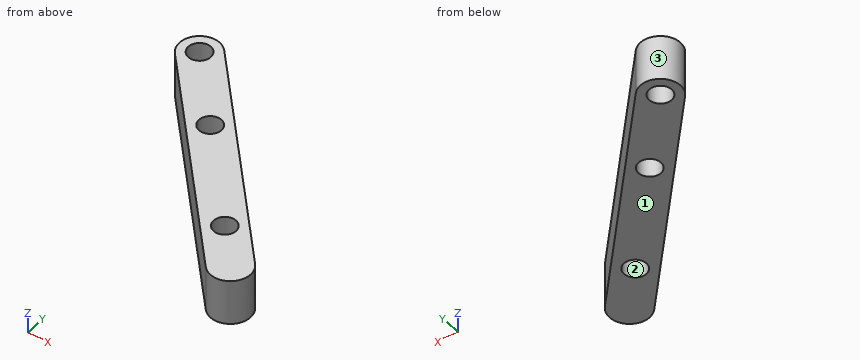
Autodesk Inventor part; units mm, degrees
ref_plane "YZ Plane" through (0, 0, 0) normal (1, 0, 0) x (0, 1, 0)
ref_plane "XZ Plane" through (0, 0, 0) normal (0, 1, 0) x (-1, 0, 0)
ref_plane "XY Plane" through (0, 0, 0) normal (0, 0, 1) x (1, 0, 0)
sketch "Sketch1" plane through (0, 0, 0) normal (0, 0, 1) x (1, 0, 0)
  circle A0 centre (20.6614, -0.7818) radius 2.25
  circle A1 centre (3.6717, 18.234) radius 2.25
  circle A2 centre (-8.6609, 32.0238) radius 2.25
  arc A3 (24.8863, -10.4155) -> (29.7342, -6.0856) centre (27.3102, -8.2505) ccw
  line L0 (27.3102, -8.2505) -> (-8.6609, 32.0238) construction
  line L1 (30.2936, -5.586) -> (-5.6776, 34.6883)
  line L2 (-11.6442, 29.3592) -> (24.3269, -10.9151)
  arc A4 (24.3269, -10.9151) -> (30.2936, -5.586) centre (27.3102, -8.2505) ccw
  arc A5 (-5.6776, 34.6883) -> (-11.6442, 29.3592) centre (-8.6609, 32.0238) ccw
  point P0 (0, 0)
  point P1 (9.3247, 11.8866)
  dimension "d0" = 8
extrude "Extrusion1" add sketch "Sketch1" along normal blind 9
scale "Scale1" factors (0.5, 0.5, 0.5) then translate (3.1707, 4.611, 2.25) bodies 1
properties part number "MassiveBone3"
The model under review builds one solid part; all positions refer to its coordinate system, in mm. Face numbers are marked on the shaded views. Coordinates: 2 decimals unless noted, no trailing zeros. Write each loop counter-clockwise with the first axis right and the second up, starting at its lowest first coordinate (ties: lowest second). Pieces come first, ordered by that corner, then holes. Notation, with made-up numbers: (28, -10.75) -> (58, -10.75) arc R18 ccw to (58, 9.25) -> close; hole circle Ø1 at (64, 31.25). An arc over 180 degrees is marked (long way). One line per item, written item: value. Start each with the question number.
Q1. The part is to be moulded in two halves that separate along Y. For the marked faces 1, 2 and 3, say which applies: +Y half, -Y half, draft (parallel to the pull), parting line (faces both ways), or undercut.
Q2. To check wall thickness, follow probe 1 along X at (y, z) = (20.5, 4.3); probe 2 along Y at (x, z) = (14.5, 4.95); probe 3 along Y at (x, z) = (13, 4.25). State the ranges of each line that lie inside material, in increasing order.
Q3. Add section A-A, the plane x = 4.25. Give the boundary of the cut face in (y, z), then the cut area to 3 significant figures.
Q4. Add section C-C, the plane y = 5. Give the boundary of the cut face in (x, z), then the cut area to 3 significant figures.
Q5. Add section D-D, the plane y = 0.5. Give the boundary of the cut face in (x, z), then the cut area to 3 significant figures.
Q6. Add section B-B, the plane z = 2.8. Count the separate pieces of the cut face and the enclosed holes in it, then the cut area to 3 significant figures.
Response:
1. face 1: draft
1. face 2: undercut
1. face 3: parting line
2. probe 1: -3.16 to -2.28, -0.04 to 1.63
2. probe 2: 0.09 to 3.7, 4.74 to 6.09
2. probe 3: 1.77 to 3.21, 5.23 to 7.77
3. outline: (11.56, 2.25) -> (12.9, 2.25) -> (12.9, 6.75) -> (11.56, 6.75) -> close; (14.56, 2.25) -> (17.57, 2.25) -> (17.57, 6.75) -> (14.56, 6.75) -> close
3. area: 19.5 mm²
4. outline: (10.11, 2.25) -> (12.69, 2.25) -> (12.69, 6.75) -> (10.11, 6.75) -> close; (14.31, 2.25) -> (15.48, 2.25) -> (15.48, 6.75) -> (14.31, 6.75) -> close
4. area: 16.8 mm²
5. outline: (14.13, 2.25) -> (18.83, 2.25) -> (18.83, 6.75) -> (14.13, 6.75) -> close
5. area: 21.1 mm²
6. separate pieces: 1
6. enclosed holes: 3
6. area: 109 mm²
